Input: part model. Units: mm. Frame: model coordinates. A direction names the side the tool comes from. Give positions to 0.01 mm unless a question says otherwise; leave off trailing zeros. Loops run counter-clockwise (first coordinate to the right, second up) from the corner with the lowest first, then second, coordinate; pieces in that order, holes last. Notation, with made-up numbers: (28, 4.5) - (46, 4.5) arc R24 cw to (46, 41.5) - close; hole circle Ø10 at (-31, 71). An arc over 180 degrees is marked (long way). Answer as a JSON object with one key per item and string values. Group by question number.
(1) Access query for faces 4 (the flat face through (7, -7, 0.397)), 5 (the cylindrical face through (-3.441, -15.497, 8.536)), 6 (the flat face through (-6, -6, 8.731)). Directions: +Z, -Z, +X, -X, +Y, -Y. A direction counts if a zero-diameter tool reaches every point of the face in a straight line with its end or side. Return the directions, or none.
(2) Material intervals for L1, parallel to Y at x = 0, z = 0.1 (3 decimals); L2, parallel to Y at x = 0, z = 0.15 (3 decimals); L3, parallel to Y at x = 0, z = 5.5, sorted ascending.
(3) Section query C-C (z = 3.25). Return loops of the section in (x, y) (1 decimal).
(4) Pin query (flat end, axial travel): P1, Ø4, axis at y = -5.5, z = 7.5, coming from the +X side; P2, Ø1, axis at y = -9.5, z = 6.5, coming from the -X side; P3, Ø12.5, axis at x = 0, y = 0, coming from the -Z side; P4, Ø4, axis at y = 6, z = 2, coming from the +X side. Return the tip coordinate at first contact, or that it passes through.
(5) Mould query, pull axis Y, two halves, no side actions, for faces 1 (the cylindrical face through (-13.858, 10.626, 4.31)), 2 (the cylindrical face through (-3.441, 15.497, 0.196)), 3 (the flat face through (13, -10, 0)). Classes: +Y half, -Y half, draft (parallel to the pull), parting line (faces both ways), or undercut.
Autodesk Inventor part; units mm, degrees
ref_plane "YZ Plane" through (0, 0, 0) normal (1, 0, 0) x (0, 1, 0)
ref_plane "XZ Plane" through (0, 0, 0) normal (0, 1, 0) x (-1, 0, 0)
ref_plane "XY Plane" through (0, 0, 0) normal (0, 0, 1) x (1, 0, 0)
sketch "Sketch1" plane through (0, 0, 0) normal (0, 0, 1) x (1, 0, 0)
  circle A0 centre (0, 0) radius 17.4625
  circle A1 centre (0, 0) radius 15.875
  circle A2 centre (0, 0) radius 7.9375
  circle A3 centre (0, 0) radius 9.525
  dimension "d0" = 34.925
  dimension "d2" = 31.75
  dimension "d3" = 15.875
  dimension "d4" = 19.05
extrude "Extrusion1" add sketch "Sketch1" along normal blind 4.3656 contours A0 | A1 | A3
extrude "Extrusion2" cut sketch "Sketch1" along normal blind 0.3969 contours A1
fillet "Fillet1" radius 0.3969 2 edges at (-17.4625, 0, 0) (-7.9375, 0, 0)
mirror "Mirror1" about plane through (0, 0, 4.3656) normal (0, 0, 1)
properties part number "R10-2RS"
Recorded:
{
 "1": {"face 4": "-Z", "face 5": "+Z", "face 6": "+Z, +X, -X, +Y, -Y"},
 "2": {"L1": "y = -17.329 to -15.875, -9.525 to -8.071, 8.071 to 9.525, 15.875 to 17.329", "L2": "y = -17.376 to -15.875, -9.525 to -8.024, 8.024 to 9.525, 15.875 to 17.376", "L3": "y = -17.46 to -7.94, 7.94 to 17.46"},
 "3": {"outline": "circle Ø34.9 at (0, 0); hole circle Ø15.9 at (0, 0)"},
 "4": {"P1": "stops at x = 17.11", "P2": "stops at x = -14.96", "P3": "passes through", "P4": "stops at x = 17"},
 "5": {"face 1": "parting line", "face 2": "undercut", "face 3": "draft"}
}
